from build123d import *

# Parameters (mm, degrees)
F0_R        = 13.97
F1_DEPTH    = 19.05
F2_T1_DEPTH = 520.7
F2_T3_DEPTH = 520.7
F3_R        = 15.24
F4_DEPTH    = 12.7


# Not quite as in the source:
# - a fillet or chamfer that OpenCascade refuses, or shapes differently, is made with other operations: its cross-section is extruded or revolved along the edge and cut away or added


with BuildPart() as f1:
    # F0 (on Right) → F1 (new body, symmetric)
    with BuildSketch(Plane.YZ):
        Polygon((143.2134641072, 335.1731732972), (111.0520780853, 355.6), (-106.8340734116, 12.545215766), (-74.6726873897, -7.8816109369), align=None)
        with Locations((118.576942247, 332.0826940597)):
            Circle(F0_R, mode=Mode.SUBTRACT)
    extrude(amount=F1_DEPTH, both=True)

    # F2: fillet of radius 22.86 on 4 edges, made by hand

    # F2_s2 → F2_t1 (cut)
    with BuildSketch(Plane(origin=(0, 223.4952640736, 351.8861527791), x_dir=(1, 0, 0), z_dir=(0, -0.5361371838, -0.8441308667))):
        with BuildLine():
            ThreePointArc((19.05, 74.0478956349), (12.3544610179, 90.2123566528), (-3.81, 96.9078956349))
            Line((-3.81, 96.9078956349), (19.05, 96.9078956349))
            Line((19.05, 96.9078956349), (19.05, 74.0478956349))
        make_face()
        with BuildLine():
            ThreePointArc((3.81, 96.9078956349), (-12.3544610179, 90.2123566528), (-19.05, 74.0478956349))
            Line((-19.05, 74.0478956349), (-19.05, 96.9078956349))
            Line((-19.05, 96.9078956349), (3.81, 96.9078956349))
        make_face()
    extrude(amount=F2_T1_DEPTH, mode=Mode.SUBTRACT)

    # F2_s4 → F2_t3 (cut)
    with BuildSketch(Plane(origin=(0, -55.6713675318, -87.6527895208), x_dir=(1, 0, 0), z_dir=(0, 0.5361371838, 0.8441308667))):
        with BuildLine():
            ThreePointArc((-3.81, -58.8078956349), (12.3544610179, -65.5034346169), (19.05, -81.6678956349))
            Line((19.05, -81.6678956349), (19.05, -58.8078956349))
            Line((19.05, -58.8078956349), (-3.81, -58.8078956349))
        make_face()
        with BuildLine():
            ThreePointArc((3.81, -58.8078956349), (-12.3544610179, -65.5034346169), (-19.05, -81.6678956349))
            Line((-19.05, -81.6678956349), (-19.05, -58.8078956349))
            Line((-19.05, -58.8078956349), (3.81, -58.8078956349))
        make_face()
    extrude(amount=F2_T3_DEPTH, mode=Mode.SUBTRACT)

    # F3 (on face) → F4 (cut, symmetric)
    with BuildSketch(Plane(origin=(0, 192.8550240193, 303.6440737462), x_dir=(1, 0, 0), z_dir=(0, 0.5361371838, 0.8441308667))):
        with Locations((0, -77.8578956349)):
            Circle(F3_R)
    extrude(amount=F4_DEPTH, both=True, mode=Mode.SUBTRACT)


solid = f1.part
Source: CAD feature listing. Evaluate the final solid. Frame: model axes, mm. Coordinates: 2 decimals unless noted, no trailing zeros. Answer in a Markdown table with one row per item. Add a question column.
Q1. Pull-direction query (Z, two-part tool) for faces 1 (the face through (12.49, 9.4, 182.81)), 2 (the face through (12.214, 27.211, 164.759)), 3 (the face through (7.032, 113.119, 348.541)); classes: pulls with the +Z half, pulls with the -Z half, needs draft (parallel to the pull), parting line crosses it, or undercut.
Q2. Contact query for flat-ended pins moving along their axis: pin 1 Ø1 at (x, z) = (4, 44) entering from +Y; pin 2 Ø6 at (x, y) = (8, 22) entering from +Z; pin 3 Ø12 at (y, z) = (-19, 82) entering from -X. Output: stop coordinate, or through.
Q3. Ray query, line 1 along Z through (x, y) = (-2.5, 48.5); line 2 along X through (y, z) = (-30, 96.5); line 3 along Y through (x, z) = (9, 227.5). Return the intervals inside material, ascending.
Computed values:
| question | item | result |
|---|---|---|
| 1 | face 1 | pulls with the +Z half |
| 1 | face 2 | pulls with the -Z half |
| 1 | face 3 | undercut |
| 2 | pin 1 | stops at y = -42.97 |
| 2 | pin 2 | stops at z = 214.9 |
| 2 | pin 3 | stops at x = -12.84 |
| 3 | line 1 | z = 187.71 to 255.46 |
| 3 | line 2 | x = -18.58 to 18.58 |
| 3 | line 3 | y = 34.34 to 70.18 |
